```python
from build123d import *

# Parameters (mm, degrees)
F0_W     = 12.7
F0_H     = 12.7
F1_DEPTH = 25.4
F2_R     = 5.5626
F3_DEPTH = 19.05
F4_W     = 2.54
F4_H     = 2.54
F5_DEPTH = 12.7
F6_R     = 1.016
F7_DEPTH = 25.4


with BuildPart() as f1:
    # F0 (on Front) → F1 (new body)
    with BuildSketch(Plane.XZ):
        Rectangle(F0_W, F0_H)
    extrude(amount=-F1_DEPTH)

    # F2 (on face) → F3 (cut)
    with BuildSketch(Plane.XZ):
        Circle(F2_R)
    extrude(amount=-F3_DEPTH, mode=Mode.SUBTRACT)

    # F4 (on face) → F5 (join)
    with BuildSketch(Plane(origin=(0, 0, -6.35), x_dir=(1, 0, 0), z_dir=(0, 0, -1))):
        with Locations((0, -19.05)):
            Rectangle(F4_W, F4_H)
    extrude(amount=F5_DEPTH)

    # F6 (on face) → F7 (cut)
    with BuildSketch(Plane(origin=(0, 20.32, 0), x_dir=(-1, 0, 0), z_dir=(0, 1, 0))):
        with Locations((0, -15.875)):
            Circle(F6_R)
    extrude(amount=-F7_DEPTH, mode=Mode.SUBTRACT)


solid = f1.part
```
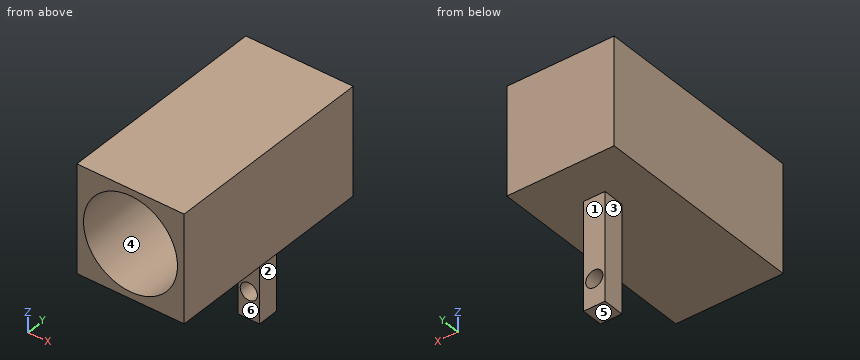
Design review of the part built by this model. Coordinates are the model's own, in mm. Face numbers are marked on the shaded views. A direction names the side the tool comes from. Round coordinates to 2 decimals unless told otherwise and drop trailing zeros. Order: outer loops, then holes, each group sorted by start corner. A loop starts at its lowest first (then second) coordinate and runs counter-clockwise, first axis right, second up. Notation, with made-up numbers: (74.5, 80) - (130.5, 80) arc R10 cw to (130.5, 94) - close; hole circle Ø4 at (37.25, 4). An arc over 180 degrees is marked (long way). Return JSON: item names as keys, results as strings.
Q1. Consider section D-D on x = 2.75. Write out the cut boundary in (y, z), plus the area to 3 significant figures.
Computed values:
{"outline": "(0, -6.35) - (25.4, -6.35) - (25.4, 6.35) - (0, 6.35) - (0, 4.84) - (19.05, 4.84) - (19.05, -4.84) - (0, -4.84) - close", "area": "138 mm2"}
Q2. The part is to be moulded in two halves that separate along Z. For the marked faces 4, 5 and 6, say which applies: pulls with the +Z half, pulls with the -Z half, needs draft (parallel to the pull), parting line crosses it, or undercut.
Computed values:
{"face 4": "undercut", "face 5": "pulls with the -Z half", "face 6": "needs draft"}
Q3. For pin 1 Ø3 at (x, z) = (0, -10) entering from +Y; pin 2 Ø5.5 at (x, z) = (-0.5, 2) entering from -Y; pin 3 Ø3 at (x, y) = (-1.5, 15.5) entering from -Z, all flat-tipped, find the tip position at first contact; note any pin that passes through.
Computed values:
{"pin 1": "stops at y = 20.32", "pin 2": "stops at y = 19.05", "pin 3": "stops at z = -6.35"}
Q4. Consider section C-C on z = 0. Write out the cut boundary in (x, y).
Computed values:
{"outline": "(-6.35, 0) - (-5.56, 0) - (-5.56, 19.05) - (5.56, 19.05) - (5.56, 0) - (6.35, 0) - (6.35, 25.4) - (-6.35, 25.4) - close"}
Q5. Consider section B-B on y = 19.75. Write out the cut boundary in (x, z) (3 decimals).
Computed values:
{"outline": "(-6.35, -6.35) - (-1.27, -6.35) - (-1.27, -19.05) - (1.27, -19.05) - (1.27, -6.35) - (6.35, -6.35) - (6.35, 6.35) - (-6.35, 6.35) - close; hole circle Ø2.032 at (0, -15.875)"}
Q6. Wall thickness on L1, parallel to Z at x = 0, y = 18.45; L2, parallel to Z at x = 0, y = 19.65; L3, parallel to Z at x = 0, y = 5.5: over which ranges is each line inside the solid? List them lowest first. Write a range as [from, to].
Computed values:
{"L1": "z = [-19.05, -16.89], [-14.86, -5.56], [5.56, 6.35]", "L2": "z = [-19.05, -16.89], [-14.86, 6.35]", "L3": "z = [-6.35, -5.56], [5.56, 6.35]"}
Q7. Consider section A-A on x = 0. Write out the cut boundary in (y, z), plus the area to 3 significant figures.
Computed values:
{"outline": "(0, -6.35) - (17.78, -6.35) - (17.78, -14.86) - (20.32, -14.86) - (20.32, -6.35) - (25.4, -6.35) - (25.4, 6.35) - (0, 6.35) - (0, 5.56) - (19.05, 5.56) - (19.05, -5.56) - (0, -5.56) - close; (17.78, -19.05) - (20.32, -19.05) - (20.32, -16.89) - (17.78, -16.89) - close", "area": "138 mm2"}
Q8. Machinability: for the marked faces 1, 2 and 3, which of the approach directions +Z, -Z, +X, -X, +Y, -Y give a long, thin tool a straight path to every point of the face, cutting with its end or side? Answer none if there is none.
Computed values:
{"face 1": "-Z, +X, -X, +Y", "face 2": "-Z, +X, +Y, -Y", "face 3": "-Z, -X, +Y, -Y"}
